For this review, take the finished solid that the model builds, in its own axes (mm). A direction names the side the tool comes from. Give positions to 0.01 mm unless a question says otherwise; leave off trailing zeros. Write each loop counter-clockwise with the first axis right and the second up, starting at its lowest first coordinate (ties: lowest second). Pieces come first, ordered by that corner, then holes. Notation, with made-up numbers: M 30,64.5 L 83,64.5 A25 ccw 83,80.5 Z; hole C 12,4.5 d3. An arc over 180 degrees is marked long. Write item = value, one per line.
```python
from build123d import *

# Parameters (mm, degrees)
BOSS_EXTRUDE1_DEPTH          = 101.6
FILLET1_R                    = 6.35
F_3_8_16_TAPPED_HOLE2_D      = 7.9375
F_3_8_16_TAPPED_HOLE2_DEPTH  = 16.002
F_3_8_16_TAPPED_HOLE2_TIP    = 2.384665582
SKETCH7_R                    = 9.525
CUT_EXTRUDE1_DEPTH           = 125.734690748
BOSS_EXTRUDE2_DEPTH          = 31.75
BOSS_EXTRUDE3_START          = -101.6
BOSS_EXTRUDE3_DEPTH          = 31.75
SKETCH9_R                    = 6.35
CUT_EXTRUDE2_DEPTH           = 3.175
F_3_8_16_TAPPED_HOLE3_REACH  = 139.938
F_3_8_16_TAPPED_HOLE3_BORE_R = 3.96875


with BuildPart() as part:
    # Sketch1 → Boss-Extrude1 (new body)
    with BuildSketch(Plane.XY):
        Polygon((0, 0), (0, 31.75), (65.024, 31.75), (65.024, 0), (58.674, 0), (58.674, 6.35), (6.35, 6.35), (6.35, 0), align=None)
    extrude(amount=-BOSS_EXTRUDE1_DEPTH)

    # Fillet1
    fillet1_edges = [part.edges().sort_by_distance(p)[0] for p in [
        (58.674, 6.35, -50.8),
        (6.35, 6.35, -50.8),
    ]]
    fillet(fillet1_edges, radius=FILLET1_R - 0.0001)  # a hair under: the kernel refuses the full size

    # 3/8-16 Tapped Hole2
    with Locations(Plane.XY):
        with Locations((31.75, 22.352)):
            Hole(F_3_8_16_TAPPED_HOLE2_D / 2, depth=F_3_8_16_TAPPED_HOLE2_DEPTH)
            with Locations((0, 0, -(F_3_8_16_TAPPED_HOLE2_DEPTH + F_3_8_16_TAPPED_HOLE2_TIP / 2))):  # 118° drill point
                Cone(0, F_3_8_16_TAPPED_HOLE2_D / 2, F_3_8_16_TAPPED_HOLE2_TIP, mode=Mode.SUBTRACT)

    # Sketch7 → Cut-Extrude1 (cut, through all)
    with BuildSketch(Plane(origin=(0, 31.75, 0), x_dir=(1, 0, 0), z_dir=(0, 1, 0))):
        with Locations(Location((32.512, 50.8, 0), (0, 0, 270))):
            Circle(SKETCH7_R)
    extrude(amount=-CUT_EXTRUDE1_DEPTH, mode=Mode.SUBTRACT)

    # Sketch8 → Boss-Extrude2 (add)
    with BuildSketch(Plane.XY):
        Polygon((14.224, 31.75), (14.224, 38.1), (7.112, 38.1), (7.112, 69.85), (13.462, 69.85), (29.21, 54.102), (29.21, 47.752), (35.814, 47.752), (35.814, 54.102), (51.562, 69.85), (57.912, 69.85), (57.912, 38.1), (50.8, 38.1), (50.8, 31.75), align=None)
    extrude(amount=-BOSS_EXTRUDE2_DEPTH)

    # Sketch8<3> → Boss-Extrude3 (add)
    with BuildSketch(Plane.XY.offset(BOSS_EXTRUDE3_START)):
        Polygon((14.224, 31.75), (14.224, 38.1), (7.112, 38.1), (7.112, 69.85), (13.462, 69.85), (29.21, 54.102), (29.21, 47.752), (35.814, 47.752), (35.814, 54.102), (51.562, 69.85), (57.912, 69.85), (57.912, 38.1), (50.8, 38.1), (50.8, 31.75), align=None)
    extrude(amount=BOSS_EXTRUDE3_DEPTH)

    # Sketch9 → Cut-Extrude2 (cut)
    with BuildSketch(Plane.ZY):
        with Locations((-50.8, 16.002)):
            Circle(SKETCH9_R)
    extrude(amount=-CUT_EXTRUDE2_DEPTH, mode=Mode.SUBTRACT)

    # 3/8-16 Tapped Hole3 bore → 3/8-16 Tapped Hole3 (cut, up to next)
    with BuildSketch(Plane.ZY.offset(-3.175), mode=Mode.PRIVATE) as f_3_8_16_tapped_hole3_sk1:
        with Locations((-50.8, 16.002)):
            Circle(F_3_8_16_TAPPED_HOLE3_BORE_R)
    f_3_8_16_tapped_hole3_tool1 = extrude(f_3_8_16_tapped_hole3_sk1.sketch, amount=-F_3_8_16_TAPPED_HOLE3_REACH, mode=Mode.PRIVATE) & part.part
    add(f_3_8_16_tapped_hole3_tool1.solids().sort_by_distance((3.175, 16.002, -50.8))[0], mode=Mode.SUBTRACT)


solid = part.part
```
1. Insertion check: P1, Ø22, axis at x = 32.512, z = -50.8, coming from the +Y side; P2, Ø8, axis at x = 12.5, z = -10, coming from the -Y side; P3, Ø10.5, axis at y = 16.002, z = -50.8, coming from the -X side (3 decimals). Each pin has a flat end and moves straight along its axis. Give the tip position at first contact, or say it passes through.
Responses:
P1 = 31.75
P2 = 4.76
P3 = 3.175
2. We need section A-A, the plane z = -50.8. Count the separate pieces of the cut face and the enclosed holes in it, then the cut area to 3 significant figures.
Responses:
separate_pieces = 3
enclosed_holes = 0
area = 1,070 mm2
3. The part is to be moulded in two halves that separate along X. For faces 1 (the face through (33, 35, -101.6)), 2 (the face through (65.024, 16, -50)), 3 (the face through (8.26, 4.54, -51.51)), 4 (the face through (29.21, 51, -86)), say which applies: +X half, -X half, draft (parallel to the pull), parting line (faces both ways), or undercut.
Responses:
face_1 = draft
face_2 = +X half
face_3 = undercut
face_4 = undercut
4. Machinability: for faces 5 (the face through (32, 47.752, -86)), 6 (the face through (7.112, 54, -16)), 7 (the face through (50.8, 35, -16)), 8 (the face through (56.9, 4.4, -51.5)), which of the approach directions +Z, -Z, +X, -X, +Y, -Y give a long, thin tool a straight path to every point of the face, cutting with its end or side? Answer none if there is none.
Responses:
face_5 = +Z, -Z, +Y
face_6 = +Z, -Z, -X, +Y
face_7 = +Z, -Z, +X
face_8 = +Z, -Z, -Y
5. We need section B-B, the plane y = 33. Write out the cut boundary in (x, z), then the cut area to 3 significant figures.
Responses:
outline = M 14.22,-101.6 L 50.8,-101.6 L 50.8,-69.85 L 14.22,-69.85 Z; M 14.22,-31.75 L 50.8,-31.75 L 50.8,0 L 14.22,0 Z
area = 2,320 mm2
6. For line 1 along Z through (x, y) = (8.5, 51.5); line 2 along X through (y, z) = (32, -8.5); line 3 along X through (y, z) = (23.25, -50.8), list the stretches that pass through material, from the lowest coordinate up. Write a range as from..to.
Responses:
line_1 = -101.6..-69.85, -31.75..0
line_2 = 14.22..50.8
line_3 = 0..22.99, 42.04..65.02
7. We need section D-D, the plane y = 64. Write out the cut boundary in (x, z).
Responses:
outline = M 7.11,-101.6 L 19.31,-101.6 L 19.31,-69.85 L 7.11,-69.85 Z; M 7.11,-31.75 L 19.31,-31.75 L 19.31,0 L 7.11,0 Z; M 45.71,-101.6 L 57.91,-101.6 L 57.91,-69.85 L 45.71,-69.85 Z; M 45.71,-31.75 L 57.91,-31.75 L 57.91,0 L 45.71,0 Z
